```python
from build123d import *

# Parameters (mm, degrees)
BOSS_EXTRUDE1_DEPTH = 3
SKETCH2_W           = 10
SKETCH2_H           = 15
BOSS_EXTRUDE2_DEPTH = 10
SKETCH4_R           = 1.75
CUT_EXTRUDE1_DEPTH  = 110.895404817
FILLET1_R           = 3
CUT_EXTRUDE4_START  = -15
SKETCH6_R           = 2.9
CUT_EXTRUDE4_DEPTH  = 11
CUT_EXTRUDE5_START  = 36
SKETCH6_2_R         = 2.9
CUT_EXTRUDE5_DEPTH  = 11
CHAMFER1_SIZE       = 1.7
SKETCH9_R           = 3.1
CUT_EXTRUDE7_DEPTH  = 1.5


with BuildPart() as part:
    # Sketch1 → Boss-Extrude1 (new body)
    with BuildSketch(Plane(origin=(0, 0, 0), x_dir=(1, 0, 0), z_dir=(0, 1, 0))):
        Polygon((59, 72), (59, 82), (0, 82), (0, 0), (59, 0), (59, 10), (72, 10), (72, 72), align=None)
    extrude(amount=BOSS_EXTRUDE1_DEPTH)

    # Sketch2 → Boss-Extrude2 (add)
    with BuildSketch(Plane.XZ):
        with Locations((67, -64.5)):
            Rectangle(SKETCH2_W, SKETCH2_H)
        with Locations((67, -17.5)):
            Rectangle(SKETCH2_W, SKETCH2_H)
    extrude(amount=BOSS_EXTRUDE2_DEPTH)

    # Sketch4 → Cut-Extrude1 (cut, through all)
    with BuildSketch(Plane(origin=(0, 3, 0), x_dir=(1, 0, 0), z_dir=(0, 1, 0))):
        with BuildLine():
            Line((4, 52), (4, 30))
            ThreePointArc((4, 30), (10.727952614, 19.727952614), (21, 13))
            Line((21, 13), (43, 13))
            ThreePointArc((43, 13), (53.272047386, 19.727952614), (60, 30))
            Line((60, 30), (60, 52))
            ThreePointArc((60, 52), (53.272047386, 62.272047386), (43, 69))
            Line((43, 69), (21, 69))
            ThreePointArc((21, 69), (10.727952614, 62.272047386), (4, 52))
        make_face()
        with Locations(Location((7, 66, 0), (0, 0, 270))):
            Circle(SKETCH4_R)
        with Locations(Location((57, 66, 0), (0, 0, 270))):
            Circle(SKETCH4_R)
        with Locations(Location((57, 16, 0), (0, 0, 270))):
            Circle(SKETCH4_R)
        with Locations(Location((7, 16, 0), (0, 0, 270))):
            Circle(SKETCH4_R)
    extrude(amount=-CUT_EXTRUDE1_DEPTH, mode=Mode.SUBTRACT)

    # Fillet1
    fillet1_edges = [part.edges().sort_by_distance(p)[0] for p in [
        (72, -10, -64.5),
        (62, -10, -64.5),
        (62, -10, -17.5),
        (72, -10, -17.5),
    ]]
    fillet(fillet1_edges, radius=FILLET1_R)

    # Sketch6 → Cut-Extrude4 (cut)
    with BuildSketch(Plane.XY.offset(-57).offset(CUT_EXTRUDE4_START)):
        with Locations(Location((66.948700041, -5, 0), (0, 0, 180))):
            Circle(SKETCH6_R)
    extrude(amount=CUT_EXTRUDE4_DEPTH, mode=Mode.SUBTRACT)

    # Sketch6<2> → Cut-Extrude5 (cut)
    with BuildSketch(Plane.XY.offset(-57).offset(CUT_EXTRUDE5_START)):
        with Locations(Location((66.948700041, -5, 0), (0, 0, 180))):
            Circle(SKETCH6_2_R)
    extrude(amount=CUT_EXTRUDE5_DEPTH, mode=Mode.SUBTRACT)

    # Chamfer1
    chamfer1_edges = [part.edges().sort_by_distance(p)[0] for p in [
        (72, 3, -41),
    ]]
    chamfer(chamfer1_edges, length=CHAMFER1_SIZE)

    # Sketch9 → Cut-Extrude7 (cut)
    with BuildSketch(Plane.XZ):
        with Locations(Location((5, -5, 0), (0, 0, 270))):
            Circle(SKETCH9_R)
        with Locations(Location((5, -77, 0), (0, 0, 270))):
            Circle(SKETCH9_R)
    extrude(amount=-CUT_EXTRUDE7_DEPTH, mode=Mode.SUBTRACT)


solid = part.part
```
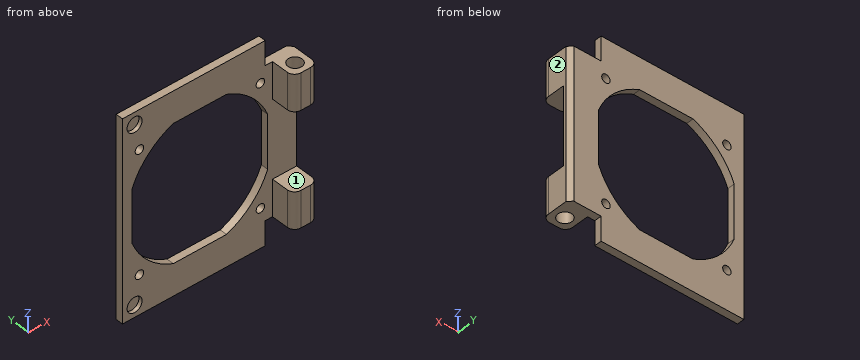
The model under review builds one solid part; all positions refer to its coordinate system, in mm. Face numbers are marked on the shaded views. Coordinates: 2 decimals unless noted, no trailing zeros. Write each loop counter-clockwise with the first axis right and the second up, starting at its lowest first coordinate (ties: lowest second). Pieces come first, ordered by that corner, then holes.
1) We need section A-A on x = 29.5. State the section outline as (y, z) points, then the cut area to 3 significant figures.
2) The part is to be moulded in two halves that separate along Z. For the marked faces 1 and 2, say which applies: pulls with the +Z half, pulls with the -Z half, needs draft (parallel to the pull), parting line crosses it, or undercut.
3) We need section D-D on x = 7. State the section outline as (y, z) points, then the cut area to 3 significant figures.
4) Clearance check with flat-ended pins moving along their axes: pin 1 Ø2 at (y, z) = (-3, -61.5) entering from -X; pin 2 Ø1.5 at (x, y) = (64, -3) entering from +Z; pin 3 Ø0.9 at (y, z) = (1, -6.5) entering from +X. State where each tip first meets the part, or that it passes through.
5) We need section B-B on y = -5. State the section outline as (x, z) points, then the cut area to 3 significant figures.
6) To check wall thickness, follow probe 1 along X at (y, z) = (0.4, -5); probe 2 along X at (y, z) = (1.8, -66); probe 3 along Y at (x, z) = (33, -78). State the ranges of each line that lie inside material, in increasing order.
7) We need section C-C on z = -16. State the section outline as (x, y) points, then the cut area to 3 significant figures.
Answer list:
1. outline: (0, -82) - (3, -82) - (3, -69) - (0, -69) - close; (0, -13) - (3, -13) - (3, 0) - (0, 0) - close
1. area: 78.0 mm2
2. face 1: undercut
2. face 2: needs draft
3. outline: (0, -82) - (3, -82) - (3, -67.75) - (0, -67.75) - (0, -74.63) - (1.5, -74.63) - (1.5, -79.37) - (0, -79.37) - close; (0, -64.25) - (3, -64.25) - (3, -57.73) - (0, -57.73) - close; (0, -24.27) - (3, -24.27) - (3, -17.75) - (0, -17.75) - close; (0, -14.25) - (3, -14.25) - (3, 0) - (0, 0) - (0, -2.63) - (1.5, -2.63) - (1.5, -7.37) - (0, -7.37) - close
3. area: 110 mm2
4. pin 1: stops at x = 62
4. pin 2: stops at z = -10
4. pin 3: stops at x = 59
5. outline: (62, -72) - (64.05, -72) - (64.05, -61) - (69.85, -61) - (69.85, -72) - (72, -72) - (72, -57) - (62, -57) - close; (62, -25) - (72, -25) - (72, -10) - (69.85, -10) - (69.85, -21) - (64.05, -21) - (64.05, -10) - (62, -10) - close
5. area: 172 mm2
6. probe 1: x = 0 to 1.9, 8.1 to 59
6. probe 2: x = 0 to 5.25, 8.75 to 15.27, 48.73 to 55.25, 58.75 to 71.5
6. probe 3: y = 0 to 3
7. outline: (0, 0) - (5.25, 0) - (5.25, 3) - (0, 3) - close; (8.75, 0) - (15.27, 0) - (15.27, 3) - (8.75, 3) - close; (48.73, 0) - (55.25, 0) - (55.25, 3) - (48.73, 3) - close; (58.75, 0) - (62, 0) - (62, -7) arc R3 ccw to (65, -10) - (69, -10) arc R3 ccw to (72, -7) - (72, 1.3) - (70.3, 3) - (58.75, 3) - close; hole circle Ø5.8 at (66.95, -5)
7. area: 163 mm2
